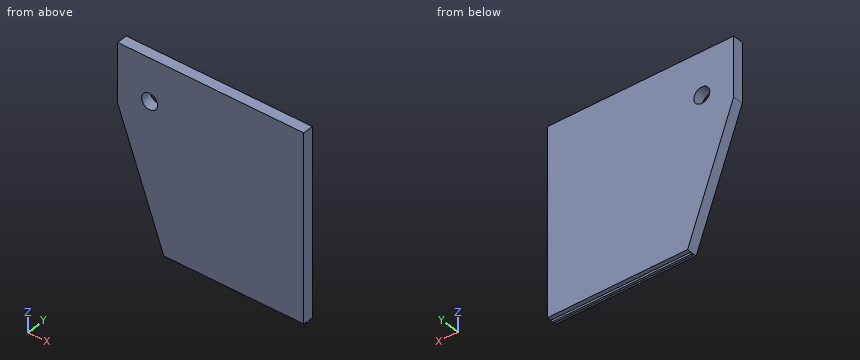
from build123d import *

# Parameters (mm, degrees)
BOSS_EXTRUDE1_DEPTH = 10
SKETCH2_W           = 131.59
SKETCH2_H           = 2
BOSS_EXTRUDE2_DEPTH = 2
SKETCH3_R           = 7.5
CUT_EXTRUDE1_DEPTH  = 250.106402969


with BuildPart() as part:
    # Sketch1 → Boss-Extrude1 (new body)
    with BuildSketch(Plane(origin=(0, 0, 0), x_dir=(1, 0, 0), z_dir=(0, 1, 0))):
        Polygon((0, 55.76), (43.41, 175), (175, 175), (175, 0), (0, 0), align=None)
    extrude(amount=BOSS_EXTRUDE1_DEPTH)

    # Sketch2 → Boss-Extrude2 (add)
    with BuildSketch(Plane(origin=(0, 0, -175), x_dir=(-1, 0, 0), z_dir=(0, 0, -1))):
        with Locations((-109.205, 5)):
            Rectangle(SKETCH2_W, SKETCH2_H)
    extrude(amount=BOSS_EXTRUDE2_DEPTH)

    # Sketch3 → Cut-Extrude1 (cut, through all)
    with BuildSketch(Plane(origin=(0, 10, 0), x_dir=(1, 0, 0), z_dir=(0, 1, 0))):
        with Locations(Location((30, 40, 0), (0, 0, 270))):
            Circle(SKETCH3_R)
    extrude(amount=-CUT_EXTRUDE1_DEPTH, mode=Mode.SUBTRACT)


solid = part.part
Build history of the part. All positions in model axes, mm. Coordinates: 2 decimals unless noted, no trailing zeros. Order: outer loops, then holes, each group sorted by start corner. A loop starts at its lowest first (then second) coordinate and runs counter-clockwise, first axis right, second up. Notation, with made-up numbers: (34, 36) - (92, 36) arc R8 ccw to (92, 42) - close; hole circle Ø9 at (73.5, -24.75). An arc over 180 degrees is marked (long way). Put each result on its own line as item: value.
1. Drop flat-ended pins along their axis: P1, Ø0.6, axis at x = 78, z = -175.5, coming from the -Y side; P2, Ø3, axis at y = 1.5, z = -102.5, coming from the -X side; P3, Ø5, axis at y = 6.5, z = -85.5, coming from the -X side. Give the stop position or say it passes through.
Answer sheet:
P1: stops at y = 4
P2: stops at x = 16.47
P3: stops at x = 9.92
2. Saw through at D-D (z = -91.5). Write the cut outline in (x, y).
Answer sheet:
outline: (13.01, 0) - (175, 0) - (175, 10) - (13.01, 10) - close
3. Saw through at A-A (z = -40). Write the cut outline in (x, y).
Answer sheet:
outline: (0, 0) - (22.5, 0) - (22.5, 10) - (0, 10) - close; (37.5, 0) - (175, 0) - (175, 10) - (37.5, 10) - close
4. Saw through at B-B (x = 30). Write the cut outline in (y, z), and give its area (3 significant figures).
Answer sheet:
outline: (0, -138.16) - (10, -138.16) - (10, -47.5) - (0, -47.5) - close; (0, -32.5) - (10, -32.5) - (10, 0) - (0, 0) - close
area: 1,230 mm^2
5. Saw through at C-C (z = -113). Write the cut outline in (x, y), and give its area (3 significant figures).
Answer sheet:
outline: (20.84, 0) - (175, 0) - (175, 10) - (20.84, 10) - close
area: 1,540 mm^2
6. Probe line 1 along X through (y, z) = (5.25, -40); line 2 along Z through (x, y) = (98.5, 9); line 3 along X through (y, z) = (6.5, -122.5). List the from-to ranges inside material, lowest first. Write a range as [from, to].
Answer sheet:
line 1: x = [0, 22.5], [37.5, 175]
line 2: z = [-175, 0]
line 3: x = [24.3, 175]
